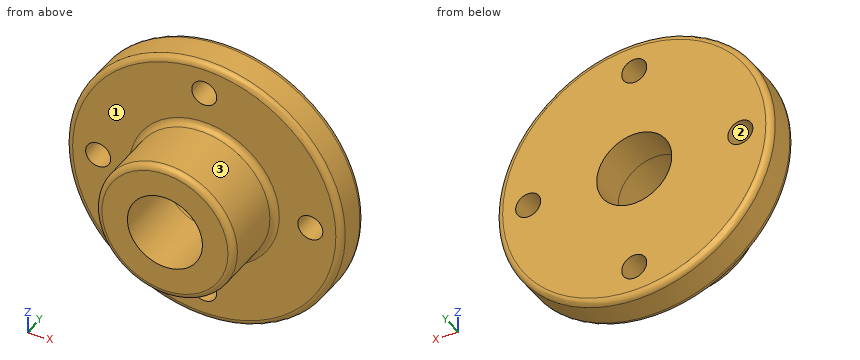
from build123d import *
from build123d import SkipClean  # not in build123d's __all__

# Parameters (mm, degrees)
F0_W            = 19.05
F0_H            = 50.8
F2_R            = 35.052
F2_R_2          = 19.05
F3_DEPTH        = 34.798
F2_R_3          = 6.35
F4_DEPTH        = 19.051
F4_COPIES_COUNT = 4
F5_R            = 3.048
F6_R            = 3.048


# Not quite as in the source:
# - after a boolean that leaves OpenCascade's solid faulty, fix() repairs it
# - a pattern or mirror of a feature is missing from the dataset's text; its kind, count and spacing are read off the source's solid


with BuildPart() as f1:
    # F0 (on Right) → F1 (revolve)
    with BuildSketch(Plane.YZ):
        with Locations((9.525, 44.45)):
            Rectangle(F0_W, F0_H)
    revolve(axis=Axis((0, 24.8311646283, 0), (0, 1, 0)))

    # F2 (on face) → F3 (join)
    with BuildSketch(Plane.XZ):
        Circle(F2_R)
        Circle(F2_R_2, mode=Mode.SUBTRACT)
    with SkipClean():  # cleaning this boolean's faces spoils the solid; the shape is the same uncleaned
        extrude(amount=F3_DEPTH)

    # F2 (on face) → F4 (cut, through all)
    with BuildSketch(Plane.XZ):
        with Locations((0, 53.848)):
            Circle(F2_R_3)
    f4 = extrude(amount=-F4_DEPTH, mode=Mode.SUBTRACT)

    add(f1.part.fix(), mode=Mode.REPLACE)

    # F4_copies: F4 ×4 about axis
    f4_copies_axis = Axis((0, 0, 0), (0, 1, 0))
    for i in range(1, F4_COPIES_COUNT):
        add(f4.rotate(f4_copies_axis, i * 360 / F4_COPIES_COUNT), clean=False, mode=Mode.SUBTRACT)

    # F5
    f5_edges = [f1.edges().sort_by_distance(p)[0] for p in [
        (0, 0, -69.85),
        (0, 19.05, -69.85),
    ]]
    fillet(f5_edges, radius=F5_R)

    # F6
    f6_edges = [f1.edges().sort_by_distance(p)[0] for p in [
        (35.052, -17.399, 0),
        (-35.052, -34.798, 0),
        (-35.052, 0, 0),
    ]]
    fillet(f6_edges, radius=F6_R)


solid = f1.part
Model file for the job. Use its own axes, mm. Face numbers are marked on the shaded views. Coordinates: 2 decimals unless noted, no trailing zeros. Order: outer loops, then holes, each group sorted by start corner. A loop starts at its lowest first (then second) coordinate and runs counter-clockwise, first axis right, second up. Notation, with made-up numbers: (28, -8.5) -> (32, -8.5) arc R33 cw to (32, 30.5) -> close; hole circle Ø3 at (56.25, 11). An arc over 180 degrees is marked (long way). Return JSON: item names as keys, results as strings. Group by question number.
Item 1: Saw through at B-B on z = 0. Write the cut outline in (x, y).
Item 2: Saw through at A-A on x = 0. Write the cut outline in (y, z).
Item 3: Saw through at C-C on y = -6. Write the cut outline in (x, z), then the cut area to 3 significant figures.
Item 4: Saw through at D-D on y = 6. Write the cut outline in (x, z).
Item 5: Wall check: line 1 along Z through (x, y) = (0, -6.5); line 2 along Y through (x, z) = (14, -53); line 3 along X through (y, z) = (6, 53.5). Give the ranges that are in metal, low to high. Write a range as [from, to].
Item 6: Pull direction X, two halves, no side cores. Call the marked faces 1, 2 and 3: pulls with the +X half, pulls with the -X half, needs draft (parallel to the pull), parting line crosses it, or undercut.
Item 7: Flat gauge pins, fed straight in: P1, Ø4, axis at y = -22, z = -30, coming from the -X side; P2, Ø20.5, axis at x = 53.848, z = 0, coming from the +Y side; P3, Ø6, axis at y = 0, z = -1.5, coming from the +X side; P4, Ø8, axis at y = -6.5, z = -17.5, coming from the +X side. Where does each tip first touch, or does it go through?
Values found:
{
 "1": {"outline": "(-69.85, 3.05) arc R3.05 ccw to (-66.8, 0) -> (-60.2, 0) -> (-60.2, 19.05) -> (-66.8, 19.05) arc R3.05 ccw to (-69.85, 16) -> close; (-47.5, 0) -> (-38.1, 0) arc R3.05 cw to (-35.05, -3.05) -> (-35.05, -31.75) arc R3.05 ccw to (-32, -34.8) -> (-19.05, -34.8) -> (-19.05, 19.05) -> (-47.5, 19.05) -> close; (19.05, -34.8) -> (32, -34.8) arc R3.05 ccw to (35.05, -31.75) -> (35.05, -3.05) arc R3.05 cw to (38.1, 0) -> (47.5, 0) -> (47.5, 19.05) -> (19.05, 19.05) -> close; (60.2, 0) -> (66.8, 0) arc R3.05 ccw to (69.85, 3.05) -> (69.85, 16) arc R3.05 ccw to (66.8, 19.05) -> (60.2, 19.05) -> close"},
 "2": {"outline": "(-34.8, -32) arc R3.05 ccw to (-31.75, -35.05) -> (-3.05, -35.05) arc R3.05 cw to (0, -38.1) -> (0, -47.5) -> (19.05, -47.5) -> (19.05, -19.05) -> (-34.8, -19.05) -> close; (-34.8, 19.05) -> (19.05, 19.05) -> (19.05, 47.5) -> (0, 47.5) -> (0, 38.1) arc R3.05 cw to (-3.05, 35.05) -> (-31.75, 35.05) arc R3.05 ccw to (-34.8, 32) -> close; (0, -66.8) arc R3.05 ccw to (3.05, -69.85) -> (16, -69.85) arc R3.05 ccw to (19.05, -66.8) -> (19.05, -60.2) -> (0, -60.2) -> close; (0, 60.2) -> (19.05, 60.2) -> (19.05, 66.8) arc R3.05 ccw to (16, 69.85) -> (3.05, 69.85) arc R3.05 ccw to (0, 66.8) -> close"},
 "3": {"outline": "circle Ø70.1 at (0, 0); hole circle Ø38.1 at (0, 0)", "area": "2,720 mm2"},
 "4": {"outline": "circle Ø139.7 at (0, 0); hole circle Ø12.7 at (-53.85, 0); hole circle Ø38.1 at (0, 0); hole circle Ø12.7 at (0, -53.85); hole circle Ø12.7 at (0, 53.85); hole circle Ø12.7 at (53.85, 0)"},
 "5": {"line 1": "z = [-35.05, -19.05], [19.05, 35.05]", "line 2": "y = [0, 19.05]", "line 3": "x = [-44.91, -6.34], [6.34, 44.91]"},
 "6": {"face 1": "needs draft", "face 2": "undercut", "face 3": "parting line crosses it"},
 "7": {"P1": "stops at x = -21.09", "P2": "stops at y = 19.05", "P3": "stops at x = 69.84", "P4": "stops at x = 32.35"}
}
